Work out the finished part from the listing and answer in its coordinate system (mm). Face numbers are marked on the shaded views. A direction names the side the tool comes from. Coordinates: 2 decimals unless noted, no trailing zeros. Loops run counter-clockwise (first coordinate to the right, second up) from the corner with the lowest first, then second, coordinate; pieces in that order, holes last. Notation, with made-up numbers: (-1, 52) -> (58, 52) arc R32 cw to (58, 88) -> close; hole circle Ø7 at (-37.75, 68.5). An arc over 180 degrees is marked (long way). Use a Markdown table: item, result.
from build123d import *

# Parameters (mm, degrees)
F0_R        = 7.5
F0_R_2      = 3
F1_DEPTH    = 15
F0_R_3      = 11
F1_FACE_R   = 7.5
F1_FACE_R_2 = 3
F2_DEPTH    = 1.5
F3_START    = 13.5
F2_FACE_R   = 11
F2_FACE_R_2 = 7.5
F3_DEPTH    = 1.5


with BuildPart() as f1:
    # F0 (on Front) → F1 (new body)
    with BuildSketch(Plane.XZ):
        Circle(F0_R)
        Circle(F0_R_2, mode=Mode.SUBTRACT)
    extrude(amount=F1_DEPTH)

    # F0 (on Front) + F1_face (on face) → F2 (join)
    with BuildSketch(Plane.XZ):
        Circle(F0_R_3)
        Circle(F0_R, mode=Mode.SUBTRACT)
    with BuildSketch(Plane.XZ.offset(15)):
        Circle(F1_FACE_R)
        Circle(F1_FACE_R_2, mode=Mode.SUBTRACT)
    extrude(amount=F2_DEPTH)

    # F2_face (on face) → F3 (join)
    with BuildSketch(Plane.XZ.offset(1.5).offset(F3_START)):
        Circle(F2_FACE_R)
        Circle(F2_FACE_R_2, mode=Mode.SUBTRACT)
    extrude(amount=F3_DEPTH)


solid = f1.part
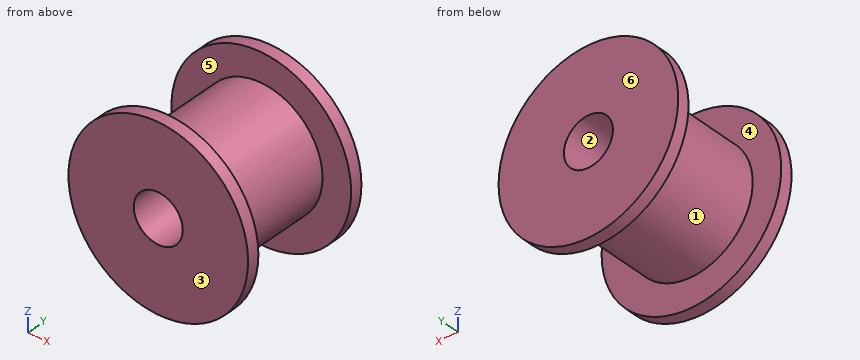
Q1. Section C-C on z = -7 is taken. Determine the outline of the cut face in (x, y).
Solved:
| item | result |
|---|---|
| outline | (-8.49, -16.5) -> (8.49, -16.5) -> (8.49, -15) -> (2.69, -15) -> (2.69, -1.5) -> (8.49, -1.5) -> (8.49, 0) -> (-8.49, 0) -> (-8.49, -1.5) -> (-2.69, -1.5) -> (-2.69, -15) -> (-8.49, -15) -> close |
Q2. Given pin 1 Ø3 at (x, y) = (5.5, -4.5) entering from +Z; pin 2 Ø6 at (x, y) = (-1, -3) entering from +Z; pin 3 Ø2 at (x, y) = (1, -4) entering from -Z; pin 4 Ø8 at (y, z) = (-8.5, 1.5) entering from -X, each flat-ended and moving along its own axis, determine where each tip first touches the part or whether it passes through.
Solved:
| item | result |
|---|---|
| pin 1 | z = 6.34 |
| pin 2 | z = 11 |
| pin 3 | z = -7.5 |
| pin 4 | x = -7.5 |
Q3. Section A-A on x = 0.75 is taken. Determine the outline of the cut face in (y, z).
Solved:
| item | result |
|---|---|
| outline | (-16.5, -10.97) -> (-15, -10.97) -> (-15, -7.46) -> (-1.5, -7.46) -> (-1.5, -10.97) -> (0, -10.97) -> (0, -2.9) -> (-16.5, -2.9) -> close; (-16.5, 2.9) -> (0, 2.9) -> (0, 10.97) -> (-1.5, 10.97) -> (-1.5, 7.46) -> (-15, 7.46) -> (-15, 10.97) -> (-16.5, 10.97) -> close |
Q4. Consider line 1 (Z direction, x = 0, y = -5.75); line 2 (Y direction, x = -1.75, z = 8.5); line 3 (X direction, y = -0.5, z = -1.5). Determine where each line is inside the solid, lowest interval first. Write a range as [from, to].
Solved:
| item | result |
|---|---|
| line 1 | [-7.5, -3], [3, 7.5] |
| line 2 | [-16.5, -15], [-1.5, 0] |
| line 3 | [-10.9, -2.6], [2.6, 10.9] |
Q5. Section D-D on x = 3.5 is taken. Determine the outline of the cut face in (y, z).
Solved:
| item | result |
|---|---|
| outline | (-16.5, -10.43) -> (-15, -10.43) -> (-15, -6.63) -> (-1.5, -6.63) -> (-1.5, -10.43) -> (0, -10.43) -> (0, 10.43) -> (-1.5, 10.43) -> (-1.5, 6.63) -> (-15, 6.63) -> (-15, 10.43) -> (-16.5, 10.43) -> close |
Q6. Determine the mould class of the marked faces 1, 2, 3 and 4 for opening direction Y: pulls with the +Y half, pulls with the -Y half, needs draft (parallel to the pull), parting line crosses it, or undercut.
Solved:
| item | result |
|---|---|
| face 1 | undercut |
| face 2 | needs draft |
| face 3 | pulls with the -Y half |
| face 4 | undercut |
Q7. For the marked faces 5 and 6, determine the directions among +Z, -Z, +X, -X, +Y, -Y from which every point of the face is accessible in a straight line to the end or side of a thin tool.
Solved:
| item | result |
|---|---|
| face 5 | none |
| face 6 | +Z, -Z, +X, -X, +Y |
Q8. Section B-B on z = 0 is taken. Determine the outline of the cut face in (x, y).
Solved:
| item | result |
|---|---|
| outline | (-11, -16.5) -> (-3, -16.5) -> (-3, 0) -> (-11, 0) -> (-11, -1.5) -> (-7.5, -1.5) -> (-7.5, -15) -> (-11, -15) -> close; (3, -16.5) -> (11, -16.5) -> (11, -15) -> (7.5, -15) -> (7.5, -1.5) -> (11, -1.5) -> (11, 0) -> (3, 0) -> close |
